Check sheet for the drawn part. Datum: minimum x, y, z corner. Units: mm. A direction names the side the tool comes from. Coordinates: 2 decimals unless noted, no trailing zeros. Loops run counter-clockwise (first coordinate to the right, second up) from the corner with the lowest first, then second, coordinate; pieces in that order, holes last.
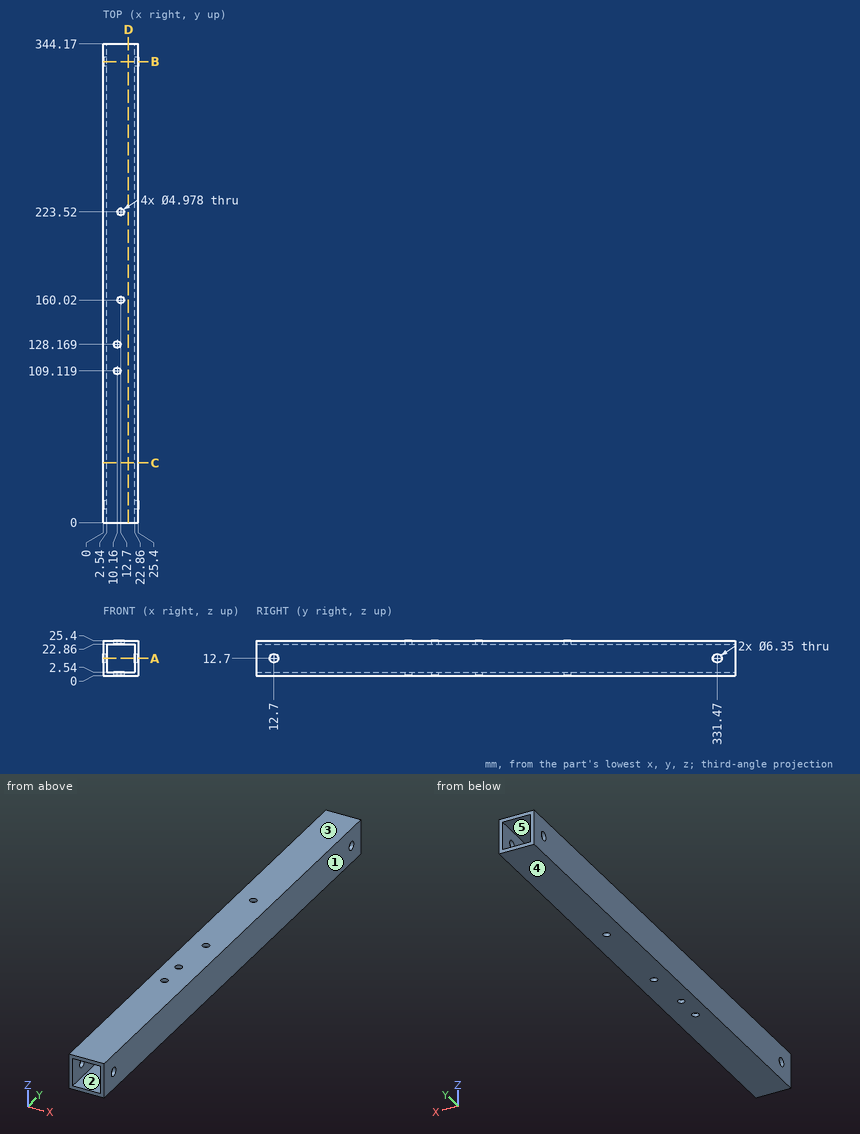
1) Set-up check for the marked faces 4 and 5: record each of +Z, -Z, +X, -X, +Y, -Y from which the full face is reachable in a straight line by a thin tool's end or side.
Answer sheet:
face 4: -Z, +X, -X, +Y, -Y
face 5: +Y, -Y
2) Depth check by flat-ended pin: pin 1 (4 mm diameter, centred on x = 12.7, y = 160.02, fed in from -Z). Enter the tip coordinate at first touch or a pass-through.
Answer sheet:
pin 1: passes through
3) Section check A-A on z = 12.7. Enter the section's corners in (x, y) (1 decimal).
Answer sheet:
outline: (0, 0) - (2.5, 0) - (2.5, 9.5) - (0, 9.5) - close; (0, 15.9) - (2.5, 15.9) - (2.5, 328.3) - (0, 328.3) - close; (0, 334.6) - (2.5, 334.6) - (2.5, 344.2) - (0, 344.2) - close; (22.9, 0) - (25.4, 0) - (25.4, 9.5) - (22.9, 9.5) - close; (22.9, 15.9) - (25.4, 15.9) - (25.4, 328.3) - (22.9, 328.3) - close; (22.9, 334.6) - (25.4, 334.6) - (25.4, 344.2) - (22.9, 344.2) - close
4) Scan lines: line 1 (Y direction, x = 10.16, z = 1); line 2 (X direction, y = 313, z = 18). Record each from-to range of solid material in increasing order.
Answer sheet:
line 1: y = 0 to 106.63, 111.61 to 125.68, 130.66 to 344.17
line 2: x = 0 to 2.54, 22.86 to 25.4
5) Section check B-B on y = 331.47. Enter the section's corners in (x, z) (1 decimal), plus the area to 3 significant figures.
Answer sheet:
outline: (0, 0) - (25.4, 0) - (25.4, 9.5) - (22.9, 9.5) - (22.9, 2.5) - (2.5, 2.5) - (2.5, 9.5) - (0, 9.5) - close; (0, 15.9) - (2.5, 15.9) - (2.5, 22.9) - (22.9, 22.9) - (22.9, 15.9) - (25.4, 15.9) - (25.4, 25.4) - (0, 25.4) - close
area: 200 mm2
6) Section check C-C on y = 43. Enter the section's corners in (x, z), plus the area to 3 significant figures.
Answer sheet:
outline: (0, 0) - (25.4, 0) - (25.4, 25.4) - (0, 25.4) - close; hole (2.54, 2.54) - (22.86, 2.54) - (22.86, 22.86) - (2.54, 22.86) - close
area: 232 mm2
7) Mould release check, pull along X, two halves, no side actions. Record for the marked faces 1, 2 and 3: +X half, -X half, draft (parallel to the pull), parting line (faces both ways), or undercut.
Answer sheet:
face 1: +X half
face 2: undercut
face 3: draft
8) Section check D-D on x = 18.25. Enter the section's corners in (y, z), plus the area to 3 significant figures.
Answer sheet:
outline: (0, 0) - (344.17, 0) - (344.17, 2.54) - (0, 2.54) - close; (0, 22.86) - (344.17, 22.86) - (344.17, 25.4) - (0, 25.4) - close
area: 1,750 mm2
